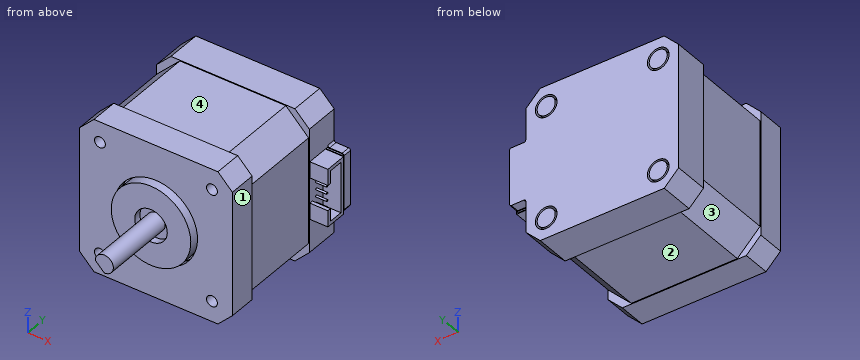
from build123d import *

# Parameters (mm, degrees)
SKETCH1_W               = 42.3
SKETCH1_H               = 42.3
BOSS_EXTRUDE1_DEPTH     = 39.25
CHAMFER1_SIZE           = 4
SKETCH2_W               = 10
SKETCH2_H               = 22.05
CUT_EXTRUDE1_DEPTH      = 1.9
MIRROR2_COPY_1_SKETCH_W = 10
MIRROR2_COPY_1_SKETCH_H = 22.05
MIRROR2_COPY_1_DEPTH    = 1.9
SKETCH3_R               = 11
BOSS_EXTRUDE2_DEPTH     = 1.9
CUT_EXTRUDE2_START      = -2
SKETCH4_R               = 11.5
SKETCH4_R_2             = 11
CUT_EXTRUDE2_DEPTH      = 2
SKETCH5_R               = 4.5
CUT_EXTRUDE3_DEPTH      = 2
SKETCH6_R               = 2.5
BOSS_EXTRUDE3_DEPTH     = 20
CUT_EXTRUDE4_START      = -15
CUT_EXTRUDE4_DEPTH      = 15
SKETCH8_R               = 1.5
CUT_EXTRUDE5_DEPTH      = 4
SKETCH10_W              = 30.925988462
SKETCH10_H              = 22.05
CUT_EXTRUDE6_DEPTH      = 0.2
CIRPATTERN1_COUNT       = 4
SKETCH11_W              = 16
SKETCH11_H              = 2.5
BOSS_EXTRUDE4_DEPTH     = 4.5
FILLET1_R               = 0.5
SKETCH12_W              = 16
SKETCH12_H              = 0.5
BOSS_EXTRUDE5_DEPTH     = 4.5
BOSS_EXTRUDE6_DEPTH     = 5
SKETCH14_R              = 0.25
BOSS_EXTRUDE7_DEPTH     = 3
SKETCH15_R              = 3
SKETCH15_R_2            = 2.5
CUT_EXTRUDE7_DEPTH      = 3


with BuildPart() as part:
    # Sketch1 → Boss-Extrude1 (new body)
    with BuildSketch(Plane(origin=(0, 0, 0), x_dir=(1, 0, 0), z_dir=(0, 1, 0))):
        Rectangle(SKETCH1_W, SKETCH1_H)
    extrude(amount=BOSS_EXTRUDE1_DEPTH)

    # Chamfer1
    chamfer1_edges = [part.edges().sort_by_distance(p)[0] for p in [
        (21.15, 19.625, 21.15),
        (-21.15, 19.625, 21.15),
        (-21.15, 19.625, -21.15),
        (21.15, 19.625, -21.15),
    ]]
    chamfer(chamfer1_edges, length=CHAMFER1_SIZE)

    # Sketch2 → Cut-Extrude1 (cut)
    with BuildSketch(Plane(origin=(19.15, 0, -19.15), x_dir=(-0.7071067811865462, 0, -0.7071067811865488), z_dir=(0.7071067811865488, 0, -0.7071067811865462))):
        with Locations((0.001572875, 18.625)):
            Rectangle(SKETCH2_W, SKETCH2_H)
    cut_extrude1 = extrude(amount=-CUT_EXTRUDE1_DEPTH, mode=Mode.SUBTRACT)

    # Mirror1: Cut-Extrude1 across plane
    add(cut_extrude1.mirror(Plane.XY), mode=Mode.SUBTRACT)

    # Mirror2: Cut-Extrude1 across plane
    add(cut_extrude1.mirror(Plane(origin=(0, 0, 0), x_dir=(0, 0, 1), z_dir=(1, 0, 0))), mode=Mode.SUBTRACT)

    # Mirror2 copy 1 sketch → Mirror2 copy 1 (cut)
    with BuildSketch(Plane(origin=(-19.15, 0, 19.15), x_dir=(0.7071067811865462, 0, 0.7071067811865488), z_dir=(-0.7071067811865488, 0, 0.7071067811865462))):
        with Locations((0.001572875, 18.625)):
            Rectangle(MIRROR2_COPY_1_SKETCH_W, MIRROR2_COPY_1_SKETCH_H)
    extrude(amount=-MIRROR2_COPY_1_DEPTH, mode=Mode.SUBTRACT)

    # Sketch3 → Boss-Extrude2 (add)
    with BuildSketch(Plane.XZ):
        with Locations(Location((0, 0, 0), (0, 0, 90))):
            Circle(SKETCH3_R)
    extrude(amount=BOSS_EXTRUDE2_DEPTH)

    # Sketch4 → Cut-Extrude2 (cut)
    with BuildSketch(Plane.XZ.offset(CUT_EXTRUDE2_START)):
        with Locations(Location((0, 0, 0), (0, 0, 270))):
            Circle(SKETCH4_R)
        with Locations(Location((0, 0, 0), (0, 0, 90))):
            Circle(SKETCH4_R_2, mode=Mode.SUBTRACT)
    extrude(amount=CUT_EXTRUDE2_DEPTH, mode=Mode.SUBTRACT)

    # Sketch5 → Cut-Extrude3 (cut)
    with BuildSketch(Plane.XZ.offset(1.9)):
        with Locations(Location((0, 0, 0), (0, 0, 270))):
            Circle(SKETCH5_R)
    extrude(amount=-CUT_EXTRUDE3_DEPTH, mode=Mode.SUBTRACT)

    # Sketch6 → Boss-Extrude3 (add)
    with BuildSketch(Plane.XZ.offset(-0.1)):
        with Locations(Location((0, 0, 0), (0, 0, 270))):
            Circle(SKETCH6_R)
    extrude(amount=BOSS_EXTRUDE3_DEPTH)

    # Sketch7 → Cut-Extrude4 (cut)
    with BuildSketch(Plane.XZ.offset(19.9).offset(CUT_EXTRUDE4_START)):
        with BuildLine():
            Line((-2.5, 0), (0, -2.5))
            ThreePointArc((0, -2.5), (-1.767766953, -1.767766953), (-2.5, 0))
        make_face()
    extrude(amount=CUT_EXTRUDE4_DEPTH, mode=Mode.SUBTRACT)

    # Sketch8 → Cut-Extrude5 (cut)
    with BuildSketch(Plane.XZ):
        with Locations(Location((-15.5, 15.5, 0), (0, 0, 270))):
            Circle(SKETCH8_R)
        with Locations(Location((15.5, 15.5, 0), (0, 0, 270))):
            Circle(SKETCH8_R)
        with Locations(Location((15.5, -15.5, 0), (0, 0, 270))):
            Circle(SKETCH8_R)
        with Locations(Location((-15.5, -15.5, 0), (0, 0, 270))):
            Circle(SKETCH8_R)
    extrude(amount=-CUT_EXTRUDE5_DEPTH, mode=Mode.SUBTRACT)

    # Sketch10 → Cut-Extrude6 (cut)
    with BuildSketch(Plane.ZY.offset(21.15)):
        with Locations((0, 18.625)):
            Rectangle(SKETCH10_W, SKETCH10_H)
    cut_extrude6 = extrude(amount=-CUT_EXTRUDE6_DEPTH, mode=Mode.SUBTRACT)

    # CirPattern1: Cut-Extrude6 ×4 about axis
    cirpattern1_axis = Axis((0, 0, 0), (0, 1, 0))
    for i in range(1, CIRPATTERN1_COUNT):
        add(cut_extrude6.rotate(cirpattern1_axis, i * 360 / CIRPATTERN1_COUNT), mode=Mode.SUBTRACT)

    # Sketch11 → Boss-Extrude4 (add)
    with BuildSketch(Plane(origin=(21.15, 0, 0), x_dir=(0, 0, -1), z_dir=(1, 0, 0))):
        with Locations((0, 38)):
            Rectangle(SKETCH11_W, SKETCH11_H)
    extrude(amount=BOSS_EXTRUDE4_DEPTH)

    # Fillet1
    fillet1_edges = [part.edges().sort_by_distance(p)[0] for p in [
        (21.15, 38, 8),
        (21.15, 38, -8),
        (25.65, 38, 8),
        (25.65, 38, -8),
    ]]
    fillet(fillet1_edges, radius=FILLET1_R)

    # Sketch12 → Boss-Extrude5 (add)
    with BuildSketch(Plane(origin=(21.15, 0, 0), x_dir=(0, 0, -1), z_dir=(1, 0, 0))):
        with Locations((0, 36.3)):
            Rectangle(SKETCH12_W, SKETCH12_H)
    extrude(amount=BOSS_EXTRUDE5_DEPTH)

    # Sketch13 → Boss-Extrude6 (add)
    with BuildSketch(Plane(origin=(21.15, 0, 0), x_dir=(0, 0, -1), z_dir=(1, 0, 0))):
        Polygon((-3.5, 30.85), (-3.5, 29.85), (-8, 29.85), (-8, 35.85), (8, 35.85), (8, 29.85), (3.5, 29.85), (3.5, 30.85), (7, 30.85), (7, 34.85), (-7, 34.85), (-7, 30.85), align=None)
    extrude(amount=BOSS_EXTRUDE6_DEPTH)

    # Sketch14 → Boss-Extrude7 (add)
    with BuildSketch(Plane(origin=(21.15, 0, 0), x_dir=(0, 0, -1), z_dir=(1, 0, 0))):
        with Locations(Location((-5, 32.35, 0), (0, 0, 180))):
            Circle(SKETCH14_R)
        with Locations(Location((-3, 32.35, 0), (0, 0, 180))):
            Circle(SKETCH14_R)
        with Locations(Location((-1, 32.35, 0), (0, 0, 180))):
            Circle(SKETCH14_R)
        with Locations(Location((1, 32.35, 0), (0, 0, 180))):
            Circle(SKETCH14_R)
        with Locations(Location((3, 32.35, 0), (0, 0, 180))):
            Circle(SKETCH14_R)
        with Locations(Location((5, 32.35, 0), (0, 0, 180))):
            Circle(SKETCH14_R)
    extrude(amount=BOSS_EXTRUDE7_DEPTH)

    # Sketch15 → Cut-Extrude7 (cut)
    # profile 1 of 4: a face of its own
    with BuildSketch(Plane(origin=(0, 39.25, 0), x_dir=(1, 0, 0), z_dir=(0, 1, 0))):
        with Locations(Location((-15.5, 15.5, 0), (0, 0, 270))):
            Circle(SKETCH15_R)
        with Locations(Location((-15.5, 15.5, 0), (0, 0, 270))):
            Circle(SKETCH15_R_2, mode=Mode.SUBTRACT)
    # profile 2 of 4: a face of its own
    with BuildSketch(Plane(origin=(0, 39.25, 0), x_dir=(1, 0, 0), z_dir=(0, 1, 0))):
        with Locations(Location((15.5, 15.5, 0), (0, 0, 270))):
            Circle(SKETCH15_R)
        with Locations(Location((15.5, 15.5, 0), (0, 0, 270))):
            Circle(SKETCH15_R_2, mode=Mode.SUBTRACT)
    # profile 3 of 4: a face of its own
    with BuildSketch(Plane(origin=(0, 39.25, 0), x_dir=(1, 0, 0), z_dir=(0, 1, 0))):
        with Locations(Location((15.5, -15.5, 0), (0, 0, 270))):
            Circle(SKETCH15_R)
        with Locations(Location((15.5, -15.5, 0), (0, 0, 270))):
            Circle(SKETCH15_R_2, mode=Mode.SUBTRACT)
    # profile 4 of 4: a face of its own
    with BuildSketch(Plane(origin=(0, 39.25, 0), x_dir=(1, 0, 0), z_dir=(0, 1, 0))):
        with Locations(Location((-15.5, -15.5, 0), (0, 0, 270))):
            Circle(SKETCH15_R)
        with Locations(Location((-15.5, -15.5, 0), (0, 0, 270))):
            Circle(SKETCH15_R_2, mode=Mode.SUBTRACT)
    extrude(amount=-CUT_EXTRUDE7_DEPTH, mode=Mode.SUBTRACT)


solid = part.part
Input: part model. Units: mm. Frame: model coordinates. Face numbers are marked on the shaded views. A direction names the side the tool comes from. Coordinates: 2 decimals unless noted, no trailing zeros. Loops run counter-clockwise (first coordinate to the right, second up) from the corner with the lowest first, then second, coordinate; pieces in that order, holes last. Notation, with made-up numbers: (-37.75, -8) -> (10.25, -8) arc R9 cw to (10.25, 0) -> close; hole circle Ø1 at (84, 40.5). An arc over 180 degrees is marked (long way). Write each question's results on one line, items separated by ' | '. Start each with the question number.
Q1. Section D-D, the plane y = -8. Return the cut outline in (x, z).
Q2. Section C-C, the plane x = 6. Return the cut outline in (y, z).
Q3. Reachability of the marked faces 1, 2, 3 and 4 from +Z, -Z, +X, -X, +Y, -Y: full face, straight path, thin tool, end or side. Return the list, or none.
Q4. Pin query (flat end, axial travel): pin 1 (1.3 mm diameter, centred on x = 23, z = -4, fed in from -Y); pin 2 (6 mm diameter, centred on x = 13.5, z = 11, fed in from -Y); pin 3 (1.2 mm diameter, centred on x = 24.5, y = 33.5, fed in from +Z). Return the tip coordinate at first contact, or that it passes through.
Q5. Ray query, line 1 (X direction, y = 1.9, z = 15.5); line 2 (Z direction, x = -15, y = 2). Return the intervals inside material, ascending. Write a range as from..to.
Q6. Section A-A, the plane y = -1. Return the cut outline in (x, z).
Q7. Section B-B, the plane y = 17.5. Return the cut outline in (x, z), plus the area to 3 significant figures.
Found:
1) outline: (-2.5, 0) -> (0, -2.5) arc R2.5 ccw (long way) to start
2) outline: (-1.9, -9.22) -> (2, -9.22) -> (2, -9.81) -> (0, -9.81) -> (0, -21.15) -> (7.6, -21.15) -> (7.6, -20.95) -> (29.65, -20.95) -> (29.65, -21.15) -> (39.25, -21.15) -> (39.25, 21.15) -> (29.65, 21.15) -> (29.65, 20.95) -> (7.6, 20.95) -> (7.6, 21.15) -> (0, 21.15) -> (0, 9.81) -> (2, 9.81) -> (2, 9.22) -> (-1.9, 9.22) -> close
3) face 1: +Z, -Z, +X, -Y | face 2: -Z, +X, -X | face 3: -Z, -X | face 4: +Z, +X, -X
4) pin 1: y = 29.85 | pin 2: y = 0 | pin 3: z = 8
5) line 1: -21.15..-17, -14..14, 17..21.15 | line 2: -21.15..-16.91, -14.09..14.09, 16.91..21.15
6) outline: circle Ø22 at (0, 0); circle Ø5 at (0, 0); hole circle Ø9 at (0, 0)
7) outline: (-20.95, -14.66) -> (-14.66, -20.95) -> (14.66, -20.95) -> (20.95, -14.66) -> (20.95, 14.66) -> (14.66, 20.95) -> (-14.66, 20.95) -> (-20.95, 14.66) -> close | area: 1,680 mm2
